The model under review builds one solid part; all positions refer to its coordinate system, in mm. A direction names the side the tool comes from. Coordinates: 2 decimals unless noted, no trailing zeros. Write each loop counter-clockwise with the first axis right and the second up, starting at its lowest first coordinate (ties: lowest second). Pieces come first, ordered by that corner, then holes.
1) Add section A-A, the plane z = -1. State the section outline as (x, y) points, then the cut area to 3 significant figures.
2) For P1, Ø3, axis at y = -1, z = -4, coming from the +X side; P2, Ø3, axis at x = 10, z = -4, coming from the +Y side; P3, Ø3, axis at x = -16.5, y = 0.5, coming from the +Z side, all flat-tipped, find the tip position at first contact; note any pin that passes through.
3) Machinability: for faces 1 (the flat face through (4, -4, -1)), 2 (the flat face through (2, -3.1, -1)), 3 (the cylindrical face through (20.26, -1.517, -5.247)), 4 (the flat face through (19.5, 1, -4)), 5 (the flat face through (-5.7, -3.5, -1.5)), which of the approach directions +Z, -Z, +X, -X, +Y, -Y give a long, thin tool a straight path to every point of the face, cutting with its end or side? Answer none if there is none.
4) Add section D-D, the plane x = 12. State the section outline as (y, z) points, then the cut area to 3 significant figures.
5) Add section B-B, the plane x = -4.5. State the section outline as (y, z) points, then the cut area to 3 significant figures.
6) For line 1 (Y direction, x = -8.5, z = -1); line 2 (Y direction, x = 20, z = -4); line 3 (Z direction, x = 14, y = 3.25), list the stretches that pass through material, from the lowest coordinate up.
7) Add section C-C, the plane z = -6.5. State the section outline as (x, y) points.
8) Mouldability with a two-part tool opening along X and no side actions: class faces 6 (the flat face through (-19.5, 2, -1)), 7 (the flat face through (21.5, 1, -3)), 8 (the flat face through (1, 0, 1)), 9 (the cylindrical face through (-16.34, 1.74, -0.76)) as released by +X, released by -X, zero draft, split by the parting line, or undercut.
from build123d import *

# Parameters (mm, degrees)
SKETCH_1_W                = 39
SKETCH_1_H                = 8
EXTRUDE_1_DEPTH           = 1
SKETCH_3_W                = 39
SKETCH_3_H                = 0.9
EXTRUDE_3_DEPTH           = 1.5
SKETCH_4_W                = 39
SKETCH_4_H                = 0.9
EXTRUDE_4_DEPTH           = 1.5
FILLET_1_R                = 4
SKETCH_5_W                = 8.5
SKETCH_5_H                = 8
EXTRUDE_5_DEPTH           = 2
SKETCH_6_W                = 8
SKETCH_6_H                = 0.9
CUT_EXTRUDE_1_DEPTH       = 1.5
FILLET_2_R                = 0.5
SKETCH_8_R                = 1.35
CUT_EXTRUDE_2_DEPTH       = 3
FILLET_3_R                = 0.5
SKETCH_9_R                = 1.1
CUT_EXTRUDE_3_DEPTH       = 3
HOLE_WIZARD_1_D           = 2.2
HOLE_WIZARD_1_DEPTH       = 7
HOLE_WIZARD_1_CSINK_D     = 4.5
HOLE_WIZARD_1_CSINK_ANGLE = 90
HOLE_WIZARD_1_TIP         = 0.660946681
EXTRUDE_6_REACH           = 24.677
SKETCH_11_R               = 1.25
FILLET_4_R                = 0.5
FILLET_5_R                = 0.5
FILLET_6_R                = 0.4
FILLET_7_R                = 0.5


with BuildPart() as part:
    # 草图1 → 凸台-拉伸1 (new body)
    with BuildSketch(Plane.XY):
        Rectangle(SKETCH_1_W, SKETCH_1_H)
    extrude(amount=EXTRUDE_1_DEPTH)

    # 草图3 → 凸台-拉伸3 (add)
    with BuildSketch(Plane(origin=(0, 0, 0), x_dir=(-1, 0, 0), z_dir=(0, 0, -1))):
        with Locations((0, -3.55)):
            Rectangle(SKETCH_3_W, SKETCH_3_H)
    extrude(amount=EXTRUDE_3_DEPTH)

    # 草图4 → 凸台-拉伸4 (add)
    with BuildSketch(Plane(origin=(0, 0, 0), x_dir=(-1, 0, 0), z_dir=(0, 0, -1))):
        with Locations((0, 3.55)):
            Rectangle(SKETCH_4_W, SKETCH_4_H)
    extrude(amount=EXTRUDE_4_DEPTH)

    # 圆角1
    fillet_1_edges = [part.edges().sort_by_distance(p)[0] for p in [
        (-19.5, -4, -0.25),
    ]]
    fillet(fillet_1_edges, radius=FILLET_1_R)

    # 草图5 → 凸台-拉伸5 (add)
    with BuildSketch(Plane(origin=(19.5, 0, 0), x_dir=(0, 0, -1), z_dir=(1, 0, 0))):
        with Locations((3.25, 0)):
            Rectangle(SKETCH_5_W, SKETCH_5_H)
    extrude(amount=EXTRUDE_5_DEPTH)

    # 草图6 → 切除-拉伸1 (cut)
    with BuildSketch(Plane(origin=(0, 0, -1.5), x_dir=(-1, 0, 0), z_dir=(0, 0, -1))):
        with Locations((-15.5, 3.55)):
            Rectangle(SKETCH_6_W, SKETCH_6_H)
    extrude(amount=-CUT_EXTRUDE_1_DEPTH, mode=Mode.SUBTRACT)

    # 圆角2
    fillet_2_edges = [part.edges().sort_by_distance(p)[0] for p in [
        (-19.5, 2, 1),
        (-18.328427125, -2.828427125, 1),
        (1, 4, 1),
        (3, -4, 1),
        (-19.5, 4, -0.25),
    ]]
    fillet(fillet_2_edges, radius=FILLET_2_R)

    # 草图8 → 切除-拉伸2 (cut)
    with BuildSketch(Plane(origin=(21.5, 0, 0), x_dir=(0, 0, -1), z_dir=(1, 0, 0))):
        with Locations((4, -1)):
            Circle(SKETCH_8_R)
    extrude(amount=-CUT_EXTRUDE_2_DEPTH, mode=Mode.SUBTRACT)

    # 圆角3
    fillet_3_edges = [part.edges().sort_by_distance(p)[0] for p in [
        (20.5, -4, -7.5),
        (20.5, 4, -7.5),
    ]]
    fillet(fillet_3_edges, radius=FILLET_3_R)

    # 草图9 → 切除-拉伸3 (cut)
    with BuildSketch(Plane(origin=(0, 0, 0), x_dir=(-1, 0, 0), z_dir=(0, 0, -1))):
        with Locations((16.5, 0.5)):
            Circle(SKETCH_9_R)
    extrude(amount=-CUT_EXTRUDE_3_DEPTH, mode=Mode.SUBTRACT)

    # 打孔尺寸(%根据)开槽沉头木螺钉的类型1
    with Locations(Plane(origin=(-16.5, 0.5, 1), x_dir=(1, 0, 0), z_dir=(0, 0, 1))):
        with Locations((0, 0)):
            CounterSinkHole(HOLE_WIZARD_1_D / 2, HOLE_WIZARD_1_CSINK_D / 2, depth=HOLE_WIZARD_1_DEPTH, counter_sink_angle=HOLE_WIZARD_1_CSINK_ANGLE)
            with Locations((0, 0, -(HOLE_WIZARD_1_DEPTH + HOLE_WIZARD_1_TIP / 2))):  # 118° drill point
                Cone(0, HOLE_WIZARD_1_D / 2, HOLE_WIZARD_1_TIP, mode=Mode.SUBTRACT)

    # 凸台-拉伸6: up to this face of the body (flat: up to its plane)
    extrude_6_end = Plane(part.part.faces().sort_by_distance((0.902646765, 0.108678474, 0))[0])
    # 草图11 → 凸台-拉伸6 (add, up to the picked face)
    with BuildSketch(Plane(origin=(0, 0, -1.5), x_dir=(-1, 0, 0), z_dir=(0, 0, -1)), mode=Mode.PRIVATE) as extrude_6_sk1:
        with BuildLine():
            Line((15, 3.1), (15, -3.1))
            Line((15, -3.1), (18.027844932, -3.1))
            ThreePointArc((18.027844932, -3.1), (19.113265817, -1.715899221), (19.5, 0))
            Line((19.5, 0), (19.5, 3.1))
            Line((19.5, 3.1), (15, 3.1))
        make_face()
        with Locations((16.5, 0.5)):
            Circle(SKETCH_11_R, mode=Mode.SUBTRACT)
    extrude_6_tool1 = split(extrude(extrude_6_sk1.sketch, amount=-EXTRUDE_6_REACH, mode=Mode.PRIVATE), bisect_by=extrude_6_end, keep=Keep.BOTH, mode=Mode.PRIVATE)
    add(extrude_6_tool1.solids().sort_by(Axis((-19.423391, 1.55, -1.5), (0, 0, 1)))[0])

    # 圆角4
    fillet_4_edges = [part.edges().sort_by_distance(p)[0] for p in [
        (-15, -3.1, -0.75),
        (-15, 3.1, -0.75),
    ]]
    fillet(fillet_4_edges, radius=FILLET_4_R)

    # 圆角5
    fillet_5_edges = [part.edges().sort_by_distance(p)[0] for p in [
        (19.5, -3.1, -0.75),
    ]]
    fillet(fillet_5_edges, radius=FILLET_5_R)

    # 圆角6
    fillet_6_edges = [part.edges().sort_by_distance(p)[0] for p in [
        (11.5, 3.1, -0.75),
        (11.5, 4, -0.75),
    ]]
    fillet(fillet_6_edges, radius=FILLET_6_R)

    # 圆角7
    fillet_7_edges = [part.edges().sort_by_distance(p)[0] for p in [
        (21.5, -1, -2.65),
        (21.5, 0, -7.5),
        (21.5, -3.853553391, -7.353553391),
        (21.5, 3.853553391, -7.353553391),
        (21.5, 0, 1),
        (21.5, 4, -3.25),
        (21.5, -4, -3.25),
        (21.5, -3.853553391, 0.853553391),
        (21.5, 3.853553391, 0.853553391),
    ]]
    fillet(fillet_7_edges, radius=FILLET_7_R)


solid = part.part
Geometry results:
1. outline: (-19.5, 0) arc R4 ccw to (-15.5, -4) - (21, -4) arc R0.5 ccw to (21.5, -3.5) - (21.5, 3.5) arc R0.5 ccw to (21, 4) - (19.5, 4) - (19.5, -2.6) arc R0.5 cw to (19, -3.1) - (-14.5, -3.1) arc R0.5 cw to (-15, -2.6) - (-15, 2.6) arc R0.5 cw to (-14.5, 3.1) - (11.1, 3.1) arc R0.4 ccw to (11.5, 3.5) - (11.5, 3.6) arc R0.4 ccw to (11.1, 4) - (-19, 4) arc R0.5 ccw to (-19.5, 3.5) - close; hole circle Ø2.5 at (-16.5, 0.5)
1. area: 98.5 mm2
2. P1: stops at x = 21.36
2. P2: passes through
2. P3: stops at z = 0.25
3. face 1: +Z, -Z, +X, -X, -Y
3. face 2: -Z
3. face 3: +X, -X
3. face 4: -Z, +Y
3. face 5: -Z, -X, +Y, -Y
4. outline: (-4, -1.5) - (-3.1, -1.5) - (-3.1, 0) - (4, 0) - (4, 0.5) arc R0.5 ccw to (3.5, 1) - (-3.5, 1) arc R0.5 ccw to (-4, 0.5) - close
4. area: 9.24 mm2
5. outline: (-4, -1.5) - (-3.1, -1.5) - (-3.1, 0) - (3.1, 0) - (3.1, -1.5) - (4, -1.5) - (4, 0.5) arc R0.5 ccw to (3.5, 1) - (-3.5, 1) arc R0.5 ccw to (-4, 0.5) - close
5. area: 10.6 mm2
6. line 1: y = -4 to -3.1, 3.1 to 4
6. line 2: y = -4 to -2.35, 0.35 to 4
6. line 3: z = 0 to 1
7. outline: (19.5, -4) - (21, -4) arc R0.5 ccw to (21.5, -3.5) - (21.5, 3.5) arc R0.5 ccw to (21, 4) - (19.5, 4) - close
8. face 6: released by -X
8. face 7: released by +X
8. face 8: zero draft
8. face 9: undercut
